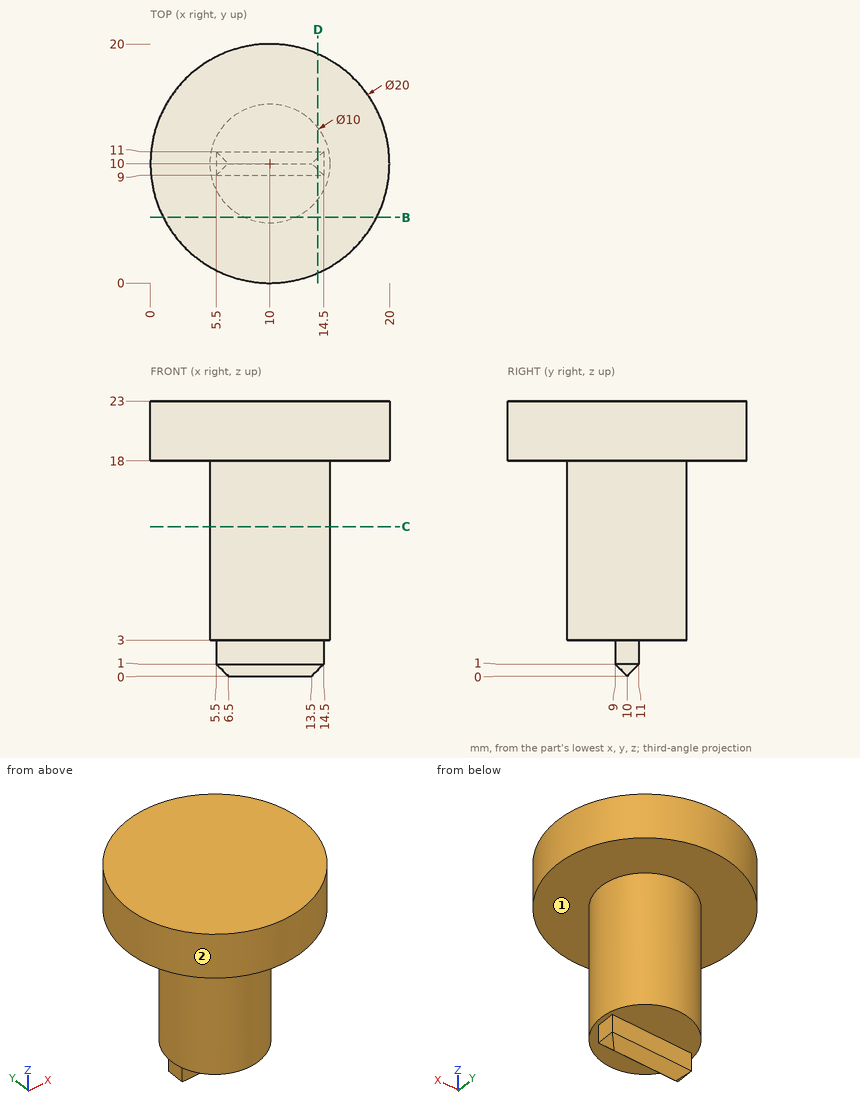
Geometry check sheet. Reference: drawing and pictorial views, mm from the part's lowest x, y, z. A direction names the side the tool comes from. Coordinates: 2 decimals unless noted, no trailing zeros. Loops run counter-clockwise (first coordinate to the right, second up) from the corner with the lowest first, then second, coordinate; pieces in that order, holes last.
1) Sectioned sample at C-C (z = 12.5). Record the boundary of the cut face in (x, y).
2) Access from +Z, -Z, +X, -X, +Y, -Y to the whole of each face (thin tool, end or side, straight path). Record for the marked faces 1 and 2.
3) Sectioned sample at D-D (x = 14). Record the boundary of the cut face in (y, z).
4) Gauge pin test, flat ends, axial feed: pin 1 (0.6 mm diameter, centred on x = 8.5, z = 2, fed in from +Y); pin 2 (1 mm diameter, centred on x = 11.5, z = 10, fed in from -Y); pin 3 (3 mm diameter, centred on x = 16, z = 19, fed in from +Y). Record the tip position at first contact, or that the pin passes through.
5) Material ranges on probe 1 along Z at (x, y) = (18.5, 7.25); probe 2 along X at (y, z) = (9.5, 2.25); probe 3 along Z at (x, y) = (9.5, 5.5), recorded low to high.
6) Sectioned sample at B-B (y = 5.5). Record the boundary of the cut face in (x, z).
Check sheet entries:
1. outline: circle Ø10 at (10, 10)
2. face 1: -Z
2. face 2: +Z, -Z
3. outline: (0.83, 18) - (7, 18) - (7, 3) - (9, 3) - (9, 1) - (9.5, 0.5) - (10.5, 0.5) - (11, 1) - (11, 3) - (13, 3) - (13, 18) - (19.17, 18) - (19.17, 23) - (0.83, 23) - close
4. pin 1: stops at y = 11
4. pin 2: stops at y = 5.1
4. pin 3: stops at y = 18.93
5. probe 1: z = 18 to 23
5. probe 2: x = 5.5 to 14.5
5. probe 3: z = 3 to 23
6. outline: (1.07, 18) - (7.82, 18) - (7.82, 3) - (12.18, 3) - (12.18, 18) - (18.93, 18) - (18.93, 23) - (1.07, 23) - close
